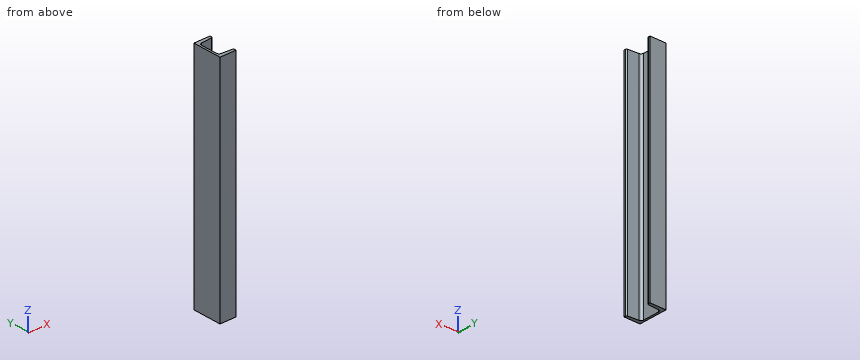
Autodesk Inventor part; units mm, degrees
ref_plane "Начальная плоскость" through (0, 0, 36) normal (0, 0, 1) x (1, 0, 0)
ref_plane "Конечная плоскость" through (0, 0, 546.459) normal (0, 0, 1) x (1, 0, 0)
ref_plane "РабПлоскость8" through (86.12, 0, 36) normal (0, 0, -1) x (-1, 0, 0)
ref_plane "Начальная плоскость" through (0, 0, 36) normal (0, 0, 1) x (1, 0, 0)
ref_plane "Конечная плоскость" through (0, 0, 546.459) normal (0, 0, 1) x (1, 0, 0)
sketch "Эскиз" plane through (0, 0, 0) normal (0, 0, 1) x (1, 0, 0)
  line L0 (36, -32.5) -> (0, -32.5)
  line L1 (36, -32.5) -> (36, -28.696)
  line L2 (33.6994, -26.2039) -> (9.9215, -24.3017)
  line L3 (4.4, -18.3208) -> (4.4, 18.3208)
  line L4 (33.6994, 26.2039) -> (9.9215, 24.3017)
  line L5 (36, 28.696) -> (36, 32.5)
  line L6 (0, 32.5) -> (36, 32.5)
  line L7 (0, -32.5) -> (0, 32.5)
  arc A0 (4.4, -18.3208) -> (9.9215, -24.3017) centre (10.4, -18.3208) ccw
  arc A1 (9.9215, 24.3017) -> (4.4, 18.3208) centre (10.4, 18.3208) ccw
  arc A2 (36, -28.696) -> (33.6994, -26.2039) centre (33.5, -28.696) ccw
  arc A3 (33.6994, 26.2039) -> (36, 28.696) centre (33.5, 28.696) ccw
  line L8 (0, 45.5) -> (0, -45.5) construction
  line L9 (-7.2974, 0) -> (43.7847, 0) construction
  point P0 (36, -26.388)
  point P1 (4.4, -23.86)
  point P2 (4.4, 23.86)
  point P3 (36, 26.388)
  dimension "d3" = 36
  dimension "d5" = 4.4
  dimension "d7" = 65
  dimension "d9" = 8.64
  dimension "d11" = 8.64
  dimension "d13" = 6.112
  dimension "d15" = 6.112
  dimension "d22" = 6
  dimension "d23" = 2.5
  dimension "d24" = 32.5
  dimension "d25" = 0
extrude "Тело" add sketch "Эскиз" along normal up to surface (510.459 mm away) from surface at 36
sketch "Sketch3" plane through (0, 0, 0) normal (0, 0, 1) x (1, 0, 0)
  line L0 (0, 0) -> (10, 0)
ref_plane "Work Plane7" through (0, 0, 0) normal (0, -1, 0) x (1, 0, 0)
sketch "Sketch4" plane through (0, 0, 0) normal (0, -1, 0) x (1, 0, 0)
  line L0 (-2, 36) -> (12, 36)
  line L1 (-2, 546.459) -> (12, 546.459)
  dimension "d29" = 510.459
ref_plane "РабПлоскость8" through (86.12, 0, 36) normal (0, 0, -1) x (-1, 0, 0)
split "Разделение1" plane through (86.12, 0, 36) removes the side toward (0, 0, -1)
equation "\"d3\" = b"
equation "\"d7\" = ParH"
equation "\"d22\" = R"
equation "\"d23\" = R1"
equation "\"d24\" = 0.5 * d7"
equation "\"d16\" = G_L"
equation "\"R1\" = 2.5"
equation "\"R\" = 6"
equation "\"t1\" = 4.4"
equation "\"t2\" = 7.2"
equation "\"ParH\" = 65"
equation "\"b\" = 36"
equation "\"msp_x1\" = 0.04 * b"
equation "\"msp_x2\" = -0.08 * t1 + 0.04 * b"
equation "\"G_L\" = d29"
equation "\"ex\" = 0"
equation "\"G_OFFSET_START\" = -36"
equation "\"G_OFFSET_END\" = 0"
equation "\"d26\" = -G_OFFSET_START"
equation "\"d27\" = G_OFFSET_END + B_L"
equation "\"B_L\" = 546.459"
properties part number "Швеллер 6.5U-510,46 ГОСТ 8240-97"
Can you work these out from the model? Positions are in its coordinate system, mm. Round coordinates to 2 decimals unless told otherwise and drop trailing zeros. Write each loop counter-clockwise with the first axis right and the second up, starting at its lowest first coordinate (ties: lowest second). Pieces come first, ordered by that corner, then holes. Notation, with made-up numbers: M 47.25,3.25 L 67.25,3.25 A7 ccw 67.25,11.25 Z; hole C 7,-39.5 d11. An arc over 180 degrees is marked long. Use a Markdown table: item, result.
Item 1: If I drill on line 1 along Y through (x, z) = (10, 465); line 2 along X through (y, z) = (-1, 413.5); line 3 along Y through (x, z) = (9, 272), over which ranges is the centre line in solid material (lowest first)? Write a range as [from, to].
Found:
| item | result |
|---|---|
| line 1 | y = [-32.5, -24.31], [24.31, 32.5] |
| line 2 | x = [0, 4.4] |
| line 3 | y = [-32.5, -24.16], [24.16, 32.5] |
Item 2: For pin 1 Ø3 at (y, z) = (-21.5, 263.5) entering from +X; pin 2 Ø4 at (y, z) = (-8, 358.5) entering from +X, each with a flat end and sliding along its axis, tell me the tip position at first contact or that it passes through.
Found:
| item | result |
|---|---|
| pin 1 | stops at x = 6.64 |
| pin 2 | stops at x = 4.4 |
Item 3: I want a section at A-A (x = 23.5). List the corners of the cut face in (y, z) for me, and give its area (3 significant figures).
Found:
| item | result |
|---|---|
| outline | M -32.5,36 L -25.39,36 L -25.39,546.46 L -32.5,546.46 Z; M 25.39,36 L 32.5,36 L 32.5,546.46 L 25.39,546.46 Z |
| area | 7,260 mm2 |
Item 4: I want a section at C-C (y = -12.5). List the corners of the cut face in (x, z) for me.
Found:
| item | result |
|---|---|
| outline | M 0,36 L 4.4,36 L 4.4,546.46 L 0,546.46 Z |
Item 5: I want a section at B-B (z = 188). List the corners of the cut face in (x, y) for me.
Found:
| item | result |
|---|---|
| outline | M 0,-32.5 L 36,-32.5 L 36,-28.7 A2.5 ccw 33.7,-26.2 L 9.92,-24.3 A6 cw 4.4,-18.32 L 4.4,18.32 A6 cw 9.92,24.3 L 33.7,26.2 A2.5 ccw 36,28.7 L 36,32.5 L 0,32.5 Z |
